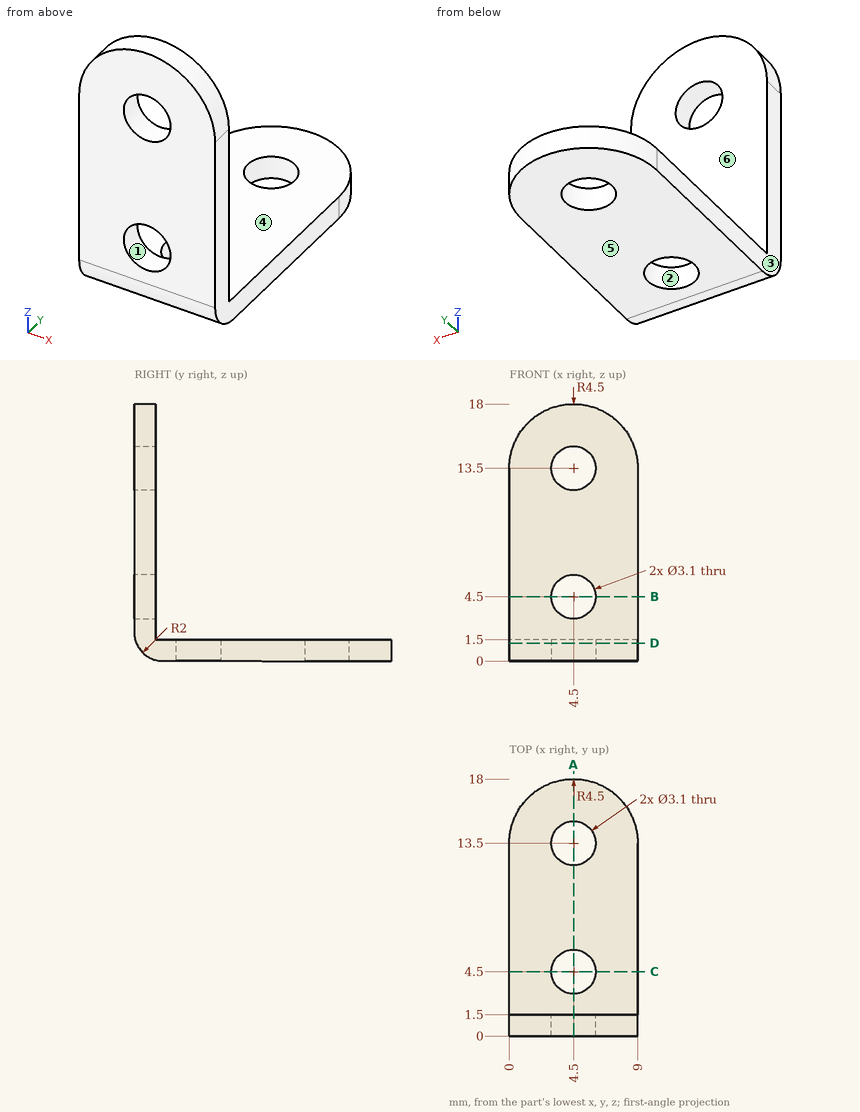
For this review, use the dimensioned drawing (mm, ordinates from the lowest corner) and the shaded views. A direction names the side the tool comes from. Coordinates: 2 decimals unless noted, no trailing zeros. Write each loop counter-clockwise with the first axis right and the second up, starting at its lowest first coordinate (ties: lowest second). Pieces come first, ordered by that corner, then holes. Notation, with made-up numbers: (13.25, 1.5) -> (45.25, 1.5) arc R24 cw to (45.25, 25.5) -> close; hole circle Ø8 at (1.25, 89.5). An arc over 180 degrees is marked (long way). Write each question's results on one line, items separated by ' | '. Start each with the question number.
(1) Take a section at A-A on x = 4.5. Write out the cut boundary in (y, z), and give its area (3 significant figures).
(2) The part is to be moulded in two halves that separate along X. For the marked faces 1, 2, 3 and 4, say which applies: pulls with the +X half, pulls with the -X half, needs draft (parallel to the pull), parting line crosses it, or undercut.
(3) Clearance check with a flat-ended pin moving along its axis: P1, Ø4.5, axis at x = 3.5, z = 7, coming from the +Y side. State where the tip first meets the part, or that it passes through.
(4) Take a section at D-D on z = 1.25. Write out the cut boundary in (x, y).
(5) Take a section at B-B on z = 4.5. Write out the cut boundary in (x, y).
(6) Tool access review of the marked faces 5 and 6: name each direction out of +Z, -Z, +X, -X, +Y, -Y from which nothing blocks a thin tool from reaching the whole face with its end or side.
(7) For line 1 along X through (y, z) = (0.9, 4.5); line 2 along Z through (x, y) = (8.5, 11), list the stretches that pass through material, from the lowest coordinate up. Write a range as from..to.
Results found:
1) outline: (0, 2) arc R2 ccw to (2, 0) -> (2.95, 0) -> (2.95, 1.5) -> (1.5, 1.5) -> (1.5, 2.95) -> (0, 2.95) -> close; (0, 6.05) -> (1.5, 6.05) -> (1.5, 11.95) -> (0, 11.95) -> close; (0, 15.05) -> (1.5, 15.05) -> (1.5, 18) -> (0, 18) -> close; (6.05, 0) -> (11.95, 0) -> (11.95, 1.5) -> (6.05, 1.5) -> close; (15.05, 0) -> (18, 0) -> (18, 1.5) -> (15.05, 1.5) -> close | area: 32.3 mm2
2) face 1: undercut | face 2: undercut | face 3: pulls with the -X half | face 4: needs draft
3) P1: stops at y = 1.5
4) outline: (0, 0.15) -> (9, 0.15) -> (9, 13.5) arc R4.5 ccw to (0, 13.5) -> close; hole circle Ø3.1 at (4.5, 4.5); hole circle Ø3.1 at (4.5, 13.5)
5) outline: (0, 0) -> (2.95, 0) -> (2.95, 1.5) -> (0, 1.5) -> close; (6.05, 0) -> (9, 0) -> (9, 1.5) -> (6.05, 1.5) -> close
6) face 5: -Z, +X, -X, +Y, -Y | face 6: +Z, +X, -X, +Y
7) line 1: x = 0..2.95, 6.05..9 | line 2: z = 0..1.5
